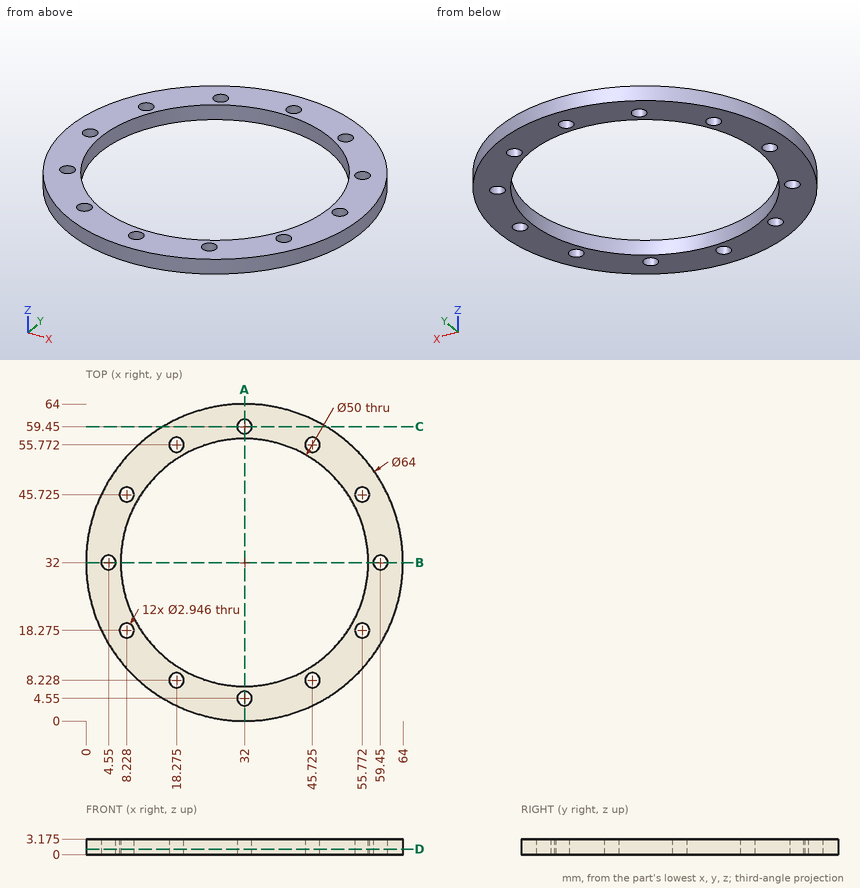
Design review of the part shown in the three views and the two pictorial views. Dimensions are in mm from the part's minimum x, y and z. Round coordinates to 2 decimals unless told otherwise and drop trailing zeros. Write each loop counter-clockwise with the first axis right and the second up, starting at its lowest first coordinate (ties: lowest second). Pieces come first, ordered by that corner, then holes. Notation, with made-up numbers: (55.5, 4.5) - (72.5, 4.5) arc R20 cw to (72.5, 36.5) - close; hole circle Ø6 at (-4, 87). An arc over 180 degrees is marked (long way). Return JSON: item names as keys, results as strings. Group by question number.
Item 1: We need section C-C on y = 59.45. Write out the cut boundary in (x, z) (1 decimal).
Item 2: Insertion check: P1, Ø1.5, axis at x = 42.5, z = 2.5, coming from the -Y side. The pin has a flat end and moves straight along its axis. Give the tip position at first contact, or say it passes through.
Item 3: For probe 1 along Y at (x, z) = (32, 0.7); probe 2 along X at (y, z) = (33, 2.75) (1 decimal); probe 3 along X at (y, z) = (23, 2.9) (1 decimal), list the stretches that pass through material, from the lowest coordinate up. Write a range as [from, to].
Item 4: We need section A-A on x = 32. Write out the cut boundary in (y, z) (1 decimal).
Item 5: We need section D-D on z = 1.15. Give the number of separate pieces and of enclosed holes in the cut face, and give its area (3 significant figures).
Model answer:
{
 "1": {"outline": "(15.6, 0) - (30.5, 0) - (30.5, 3.2) - (15.6, 3.2) - close; (33.5, 0) - (48.4, 0) - (48.4, 3.2) - (33.5, 3.2) - close"},
 "2": {"P1": "stops at y = 1.52"},
 "3": {"probe 1": "y = [0, 3.08], [6.02, 7], [57, 57.98], [60.92, 64]", "probe 2": "x = [0, 3.5], [5.6, 7], [57, 58.4], [60.5, 64]", "probe 3": "x = [1.3, 8.7], [55.3, 62.7]"},
 "4": {"outline": "(0, 0) - (3.1, 0) - (3.1, 3.2) - (0, 3.2) - close; (6, 0) - (7, 0) - (7, 3.2) - (6, 3.2) - close; (57, 0) - (58, 0) - (58, 3.2) - (57, 3.2) - close; (60.9, 0) - (64, 0) - (64, 3.2) - (60.9, 3.2) - close"},
 "5": {"separate pieces": "1", "enclosed holes": "13", "area": "1,170 mm²"}
}
